Source: CAD feature listing. Evaluate the final solid. Frame: model axes, mm. A direction names the side the tool comes from. Round coordinates to 2 decimals unless told otherwise and drop trailing zeros. Write each loop counter-clockwise with the first axis right and the second up, starting at its lowest first coordinate (ties: lowest second). Pieces come first, ordered by that corner, then holes. Notation, with made-up numbers: (51, 25) - (71, 25) arc R7 ccw to (71, 30) - close; hole circle Ø10 at (21.5, 81). An arc over 180 degrees is marked (long way). Write item = value, one per line. Start each with the question number.
```python
from build123d import *

# Parameters (mm, degrees)
SKETCH_1_R          = 2.78
SKETCH_1_R_2        = 2
EXTRUDE_1_DEPTH     = 6.35
CUT_EXTRUDE_START   = -4.83
CUT_EXTRUDE_1_DEPTH = 4.83
CHAMFER_1_SIZE      = 0.2


with BuildPart() as part:
    # 草图1 → 凸台-拉伸1 (new body)
    with BuildSketch(Plane(origin=(0, 0, 0), x_dir=(1, 0, 0), z_dir=(0, 1, 0))):
        with Locations(Location((0, 0, 0), (0, 0, 270))):
            Circle(SKETCH_1_R)
        with Locations(Location((0, 0, 0), (0, 0, 270))):
            Circle(SKETCH_1_R_2, mode=Mode.SUBTRACT)
    extrude(amount=EXTRUDE_1_DEPTH)

    # 草图2 → 切除-拉伸1 (cut)
    with BuildSketch(Plane(origin=(0, 6.35, 0), x_dir=(1, 0, 0), z_dir=(0, 1, 0)).offset(CUT_EXTRUDE_START)):
        with BuildLine():
            Line((-2.714479692, 0.6), (2.714479692, 0.6))
            ThreePointArc((2.714479692, 0.6), (2.78, 0), (2.714479692, -0.6))
            Line((2.714479692, -0.6), (-2.714479692, -0.6))
            ThreePointArc((-2.714479692, -0.6), (-2.78, 0), (-2.714479692, 0.6))
        make_face()
    extrude(amount=CUT_EXTRUDE_1_DEPTH, mode=Mode.SUBTRACT)

    # 倒角1
    chamfer_1_edges = [part.edges().sort_by_distance(p)[0] for p in [
        (-1.183215957, 6.35, 1.61245155),
        (0, 0, -2),
        (0, 6.35, -2),
    ]]
    chamfer(chamfer_1_edges, length=CHAMFER_1_SIZE)


solid = part.part
```
(1) Section A-A (z = 0). Return the cut outline in (x, y), plus the area to 3 significant figures.
(2) Section C-C (y = 5.25). Return the cut outline in (x, z), plus the area to 3 significant figures.
(3) Ray query, L1, parallel to Z at x = 0.1, y = 0.75; L2, parallel to Z at x = -0.6, y = 3; L3, parallel to X at y = 2, z = 0.8. Return the intervals inside material, ascending. Write a range as from..to.
(4) Contact query for flat-ended pins moving along their axis: P1, Ø1.5, axis at x = -1, y = 1.5, coming from the +Z side; P2, Ø1.5, axis at y = 3, z = -0.5, coming from the +X side; P3, Ø1, axis at x = 1.5, y = 5.5, coming from the +Z side. Output: stop coordinate, or through.
(5) Section B-B (x = 0). Return the cut outline in (y, z), plus the area to 3 significant figures.
(6) Reachability of faces 1 (the flat face through (0, 6.35, -2.4)), 2 (the flat face through (-2.3, 3.9, 0.6)) from +Z, -Z, +X, -X, +Y, -Y: full face, straight path, thin tool, end or side. Return the list, or none.
(7) Pull-direction query (X, two-part tool) for faces 3 (the cylindrical face through (-2.47, 3.13, 1.28)), 4 (the cylindrical face through (-0.766, 3.133, 1.847)), 5 (the flat face through (-2.3, 3.9, -0.6)); classes: +X half, -X half, draft (parallel to the pull), parting line (faces both ways), or undercut.
Solution:
q1.outline = (-2.78, 0) - (-2.2, 0) - (-2, 0.2) - (-2, 1.52) - (-2.78, 1.52) - close; (2, 0.2) - (2.2, 0) - (2.78, 0) - (2.78, 1.52) - (2, 1.52) - close
q1.area = 2.33 mm^2
q2.outline = (-2.71, -0.6) arc R2.78 ccw to (2.71, -0.6) - (1.91, -0.6) arc R2 cw to (-1.91, -0.6) - close; (-2.71, 0.6) - (-1.91, 0.6) arc R2 cw to (1.91, 0.6) - (2.71, 0.6) arc R2.78 ccw to start
q2.area = 9.82 mm^2
q3.L1 = -2.78..-2, 2..2.78
q3.L2 = -2.71..-1.91, 1.91..2.71
q3.L3 = -2.66..-1.83, 1.83..2.66
q4.P1 = 2.77
q4.P2 = 2.71
q4.P3 = 2.59
q5.outline = (0, -2.78) - (6.35, -2.78) - (6.35, -2.2) - (6.15, -2) - (0.2, -2) - (0, -2.2) - close; (0, 2.2) - (0.2, 2) - (6.15, 2) - (6.35, 2.2) - (6.35, 2.78) - (0, 2.78) - close
q5.area = 9.83 mm^2
q6.face_1 = +Z, -Z, +X, -X, +Y
q6.face_2 = +X, -X, +Y
q7.face_3 = parting line
q7.face_4 = undercut
q7.face_5 = draft
